```python
from build123d import *

# Parameters (mm, degrees)
SKETCH_1_W               = 20
SKETCH_1_H               = 20
EXTRUDE_1_DEPTH          = 34
SKETCH_2_R               = 8
EXTRUDE_2_DEPTH          = 1.5
SKETCH_3_R               = 2
EXTRUDE_3_DEPTH          = 18.4
SKETCH_4_R               = 1
CUT_EXTRUDE_1_DEPTH      = 42.263223045
MIRROR_2_COPY_1_SKETCH_R = 1
MIRROR_2_COPY_1_DEPTH    = 42.263223045
FILLET_2_R               = 2


with BuildPart() as part:
    # 草圖1 → 填料-伸長1 (new body)
    with BuildSketch(Plane.XY):
        with Locations((-11.134180278, 0)):
            Rectangle(SKETCH_1_W, SKETCH_1_H)
    extrude(amount=EXTRUDE_1_DEPTH)

    # 草圖2 → 填料-伸長2 (add)
    with BuildSketch(Plane.XY.offset(34)):
        with Locations((-11.134180278, 0)):
            Circle(SKETCH_2_R)
    extrude(amount=EXTRUDE_2_DEPTH)

    # 草圖3 → 填料-伸長3 (add)
    with BuildSketch(Plane.XY.offset(35.5)):
        with Locations((-11.134180278, 0)):
            Circle(SKETCH_3_R)
    extrude(amount=EXTRUDE_3_DEPTH)

    # 草圖4 → 除料-伸長1 (cut, through all)
    with BuildSketch(Plane.XY.offset(34)):
        with Locations((-18.634180278, 7.5)):
            Circle(SKETCH_4_R)
    cut_extrude_1 = extrude(amount=-CUT_EXTRUDE_1_DEPTH, mode=Mode.SUBTRACT)

    # 鏡射1: 除料-伸長1 across plane
    add(cut_extrude_1.mirror(Plane.ZY.offset(11.134180278)), mode=Mode.SUBTRACT)

    # 鏡射2: 除料-伸長1 across plane
    add(cut_extrude_1.mirror(Plane(origin=(0, 0, 0), x_dir=(0, 0, 1), z_dir=(0, -1, 0))), mode=Mode.SUBTRACT)

    # 鏡射2 copy 1 sketch → 鏡射2 copy 1 (cut, through all)
    with BuildSketch(Plane(origin=(-22.268360557, 0, 34), x_dir=(-1, 0, 0), z_dir=(0, 0, 1))):
        with Locations((-18.634180278, 7.5)):
            Circle(MIRROR_2_COPY_1_SKETCH_R)
    extrude(amount=-MIRROR_2_COPY_1_DEPTH, mode=Mode.SUBTRACT)

    # 圓角2
    fillet_2_edges = [part.edges().sort_by_distance(p)[0] for p in [
        (-21.134180278, 10, 17),
        (-1.134180278, 10, 17),
        (-1.134180278, -10, 17),
        (-21.134180278, -10, 17),
    ]]
    fillet(fillet_2_edges, radius=FILLET_2_R)


solid = part.part
```
Check sheet for the modelled part. Datum: model origin and axes. Units: mm. A direction names the side the tool comes from. Give positions to 0.01 mm unless a question says otherwise; leave off trailing zeros. Order: outer loops, then holes, each group sorted by start corner. A loop starts at its lowest first (then second) coordinate and runs counter-clockwise, first axis right, second up. Notation, with made-up numbers: (-27.5, 42.25) -> (21.5, 42.25) arc R17 ccw to (21.5, 70.25) -> close; hole circle Ø9 at (45.25, 19.25). An arc over 180 degrees is marked (long way). Return JSON: item names as keys, results as strings.
1. Cross-section at D-D, the plane x = -8. Record the cut outline in (y, z), plus the area to 3 significant figures.
From the geometry:
{"outline": "(-10, 0) -> (10, 0) -> (10, 34) -> (7.36, 34) -> (7.36, 35.5) -> (-7.36, 35.5) -> (-7.36, 34) -> (-10, 34) -> close", "area": "702 mm^2"}
2. Set-up check for faces 1 (the cylindrical face through (-9.3, -0.8, 44.6)), 2 (the flat face through (-1.134, 0, 17)): record each of +Z, -Z, +X, -X, +Y, -Y from which the full face is reachable in a straight line by a thin tool's end or side.
From the geometry:
{"face 1": "+Z", "face 2": "+Z, -Z, +X, +Y, -Y"}
3. Mould release check, pull along Y, two halves, no side actions. Record for faces 3 (the flat face through (-18, 5, 34)), 4 (the cylindrical face through (-1.736, 9.43, 17.238)), 5 (the cylindrical face through (-3.5, -8.49, 17.24)), 6 (the cylindrical face through (-17.68, -7.8, 17.24)): +Y half, -Y half, draft (parallel to the pull), parting line (faces both ways), or undercut.
From the geometry:
{"face 3": "draft", "face 4": "+Y half", "face 5": "undercut", "face 6": "undercut"}
4. Go/stop test with flat-tipped pins: P1, Ø5, axis at x = -16.5, y = 0, coming from the +Z side; P2, Ø6, axis at x = -14, y = -1.5, coming from the +Z side; P3, Ø2.5, axis at x = -3.63, y = 7.5, coming from the +Z side; P4, Ø6, axis at y = 0, z = 44.5, coming from the +X side. Record where each tip stops, or that it passes through.
From the geometry:
{"P1": "z = 35.5", "P2": "z = 53.9", "P3": "z = 34", "P4": "x = -9.13"}
5. Cross-section at A-A, the plane z = 24. Record the cut outline in (x, y).
From the geometry:
{"outline": "(-21.13, -8) arc R2 ccw to (-19.13, -10) -> (-3.13, -10) arc R2 ccw to (-1.13, -8) -> (-1.13, 8) arc R2 ccw to (-3.13, 10) -> (-19.13, 10) arc R2 ccw to (-21.13, 8) -> close; hole circle Ø2 at (-18.63, -7.5); hole circle Ø2 at (-18.63, 7.5); hole circle Ø2 at (-3.63, -7.5); hole circle Ø2 at (-3.63, 7.5)"}
6. Material ranges on probe 1 along X at (y, z) = (-7.5, 26.5); probe 2 along Z at (x, y) = (-8.75, -2.5); probe 3 along Y at (x, z) = (-11.25, 44.5), recorded low to high. Write a range as [from, to].
From the geometry:
{"probe 1": "[-21.13, -19.63], [-17.63, -4.63], [-2.63, -1.13]", "probe 2": "[0, 35.5]", "probe 3": "[-2, 2]"}
7. Cross-section at C-C, the plane y = -7.5. Record the cut outline in (x, z), plus the area to 3 significant figures.
From the geometry:
{"outline": "(-21.13, 0) -> (-19.63, 0) -> (-19.63, 34) -> (-21.13, 34) -> close; (-17.63, 0) -> (-4.63, 0) -> (-4.63, 34) -> (-8.35, 34) -> (-8.35, 35.5) -> (-13.92, 35.5) -> (-13.92, 34) -> (-17.63, 34) -> close; (-2.63, 0) -> (-1.13, 0) -> (-1.13, 34) -> (-2.63, 34) -> close", "area": "552 mm^2"}
8. Cross-section at B-B, the plane y = 0. Record the cut outline in (x, z), plus the area to 3 significant figures.
From the geometry:
{"outline": "(-21.13, 0) -> (-1.13, 0) -> (-1.13, 34) -> (-3.13, 34) -> (-3.13, 35.5) -> (-9.13, 35.5) -> (-9.13, 53.9) -> (-13.13, 53.9) -> (-13.13, 35.5) -> (-19.13, 35.5) -> (-19.13, 34) -> (-21.13, 34) -> close", "area": "778 mm^2"}
